Source: CAD feature listing. Evaluate the final solid. Frame: model axes, mm. A direction names the side the tool comes from. Coordinates: 2 decimals unless noted, no trailing zeros. Write each loop counter-clockwise with the first axis right and the second up, starting at its lowest first coordinate (ties: lowest second). Pieces come first, ordered by that corner, then holes. Notation, with made-up numbers: (-1.5, 68.5) -> (50.5, 68.5) arc R23 cw to (50.5, 85.5) -> close; hole circle Ø6 at (66.5, -18.5). An arc over 180 degrees is marked (long way). One line per item, written item: value. Start each with the question number.
1. Section query A-A, the plane z = 4.5. Output: boundary loops of the cut face in (x, y), and give its area (3 significant figures).
2. Line query: line 1 (Y direction, x = 0, z = 4); line 2 (X direction, y = 2.75, z = 3.75); line 3 (Y direction, x = -0.25, z = 5.25). Output: solid intervals per line, ascending.
3. Mould query, pull axis X, two halves, no side actions, for faces 5 (the cylindrical face through (-3, 0, 3)), 6 (the flat face through (4.267, -2.51, 2.465)), 7 (the flat face through (2.5, 2.3, 0)). Classes: released by +X, released by -X, zero draft, split by the parting line, or undercut.
4. Access query for faces 1 (the flat face through (0.4, -5.3, 5)), 2 (the flat face through (-4.307, -2.44, 2.465)), 3 (the flat face through (4.307, 2.44, 2.465)), 4 (the flat face through (0, -4.95, 2)). Directions: +Z, -Z, +X, -X, +Y, -Y. A direction counts if a zero-diameter tool reaches every point of the face in a straight line with its end or side. Return the directions, or none.
5. Section query B-B, the plane x = 0. Output: boundary loops of the cut face in (y, z) (3 decimals).
6. Section query D-D, the plane y = 3.5. Output: boundary loops of the cut face in (x, z), and give its area (3 significant figures).
7. Section query C-C, the plane y = 2.25. Output: boundary loops of the cut face in (x, z).
from build123d import *

# Parameters (mm, degrees)
SKETCH1_R           = 3
BOSS_EXTRUDE1_DEPTH = 5
SKETCH2_R           = 5.975
SKETCH2_R_2         = 3
BOSS_EXTRUDE2_DEPTH = 1.5


with BuildPart() as part:
    # Sketch1 → Boss-Extrude1 (new body)
    with BuildSketch(Plane.XY):
        Polygon((-5.715767665, 0), (-2.857883832, -4.95), (2.857883832, -4.95), (5.715767665, 0), (2.857883832, 4.95), (-2.857883832, 4.95), align=None)
        Circle(SKETCH1_R, mode=Mode.SUBTRACT)
    extrude(amount=BOSS_EXTRUDE1_DEPTH)

    # Sketch2 → Boss-Extrude2 (add)
    with BuildSketch(Plane.XY.offset(5)):
        Circle(SKETCH2_R)
        Circle(SKETCH2_R_2, mode=Mode.SUBTRACT)
    extrude(amount=BOSS_EXTRUDE2_DEPTH)


solid = part.part
Computed values:
1. outline: (-5.72, 0) -> (-2.86, -4.95) -> (2.86, -4.95) -> (5.72, 0) -> (2.86, 4.95) -> (-2.86, 4.95) -> close; hole circle Ø6 at (0, 0)
1. area: 56.6 mm²
2. line 1: y = -4.95 to -3, 3 to 4.95
2. line 2: x = -4.13 to -1.2, 1.2 to 4.13
2. line 3: y = -5.97 to -2.99, 2.99 to 5.97
3. face 5: undercut
3. face 6: released by +X
3. face 7: zero draft
4. face 1: -Z
4. face 2: -Z, -X, -Y
4. face 3: -Z, +X, +Y
4. face 4: -Z, +X, -X, -Y
5. outline: (-5.975, 5) -> (-4.95, 5) -> (-4.95, 0) -> (-3, 0) -> (-3, 6.5) -> (-5.975, 6.5) -> close; (3, 0) -> (4.95, 0) -> (4.95, 5) -> (5.975, 5) -> (5.975, 6.5) -> (3, 6.5) -> close
6. outline: (-4.84, 5) -> (-3.7, 5) -> (-3.7, 0) -> (3.7, 0) -> (3.7, 5) -> (4.84, 5) -> (4.84, 6.5) -> (-4.84, 6.5) -> close
6. area: 51.5 mm²
7. outline: (-5.54, 5) -> (-4.42, 5) -> (-4.42, 0) -> (-1.98, 0) -> (-1.98, 6.5) -> (-5.54, 6.5) -> close; (1.98, 0) -> (4.42, 0) -> (4.42, 5) -> (5.54, 5) -> (5.54, 6.5) -> (1.98, 6.5) -> close
